Geometry: final body of the model. Coordinates: model frame, mm. A direction names the side the tool comes from. Give positions to 0.01 mm unless a question says otherwise; leave off trailing zeros. Write each loop counter-clockwise with the first axis right and the second up, starting at its lowest first coordinate (ties: lowest second). Pieces come first, ordered by that corner, then holes. Notation, with made-up numbers: (88, 0.5) - (119, 0.5) arc R21 ccw to (119, 25.5) - close; hole circle Ø8 at (36.5, -38.5). An arc over 180 degrees is marked (long way). Use CSV: the item, a comma, the result in double quotes. Start each with the question number.
(1) Section A-A on x = 6. Output: boundary loops of the cut face in (y, z), and give its area (3 significant figures).
(2) Reachability of faces 4 (the flat face through (10, 4, -10)), 5 (the flat face through (28.63, 3.45, -7.57)), 6 (the flat face through (28, 11, -10)) from +Z, -Z, +X, -X, +Y, -Y: full face, straight path, thin tool, end or side. Return the list, or none.
(3) Draft query along X for faces 1 (the flat face through (20, 0, -10)), 2 (the flat face through (20, 7, -10)), 3 (the flat face through (31.413, 3.451, -7.597)). Return one class per face: released by +X, released by -X, zero draft, split by the parting line, or undercut.
(4) Section B-B on y = 5.5. Output: boundary loops of the cut face in (x, z).
(5) Section C-C on z = -10. Output: boundary loops of the cut face in (x, y), and give its area (3 significant figures).
(6) Section D-D on y = 1.75. Output: boundary loops of the cut face in (x, z), and give its area (3 significant figures).
(7) Line query: probe 1 along X at (y, z) = (1.8, -10); probe 2 along X at (y, z) = (5, -10.5); probe 3 along Z at (x, y) = (6, 2.85). Output: solid intervals per line, ascending. Write a range as [from, to].
(8) First-contact query: pin 1 Ø1 at (y, z) = (6.5, -13) entering from -X; pin 2 Ø4.5 at (x, z) = (30, -10) entering from +Y; pin 3 Ø6 at (x, z) = (8.5, -11) entering from +Y; pin 4 Ø3 at (x, z) = (30.5, -11) entering from -Y. Flat tips, straight axial feed; report the tip coordinate or a pass-through.
from build123d import *

# Parameters (mm, degrees)
SKETCH1_W           = 40
SKETCH1_H           = 20
SKETCH1_R           = 2.75
BOSS_EXTRUDE1_DEPTH = 4
SKETCH2_W           = 20
SKETCH2_H           = 20
BOSS_EXTRUDE2_DEPTH = 7
SKETCH3_R           = 1.75
CUT_EXTRUDE1_DEPTH  = 12
CUT_EXTRUDE2_DEPTH  = 7


with BuildPart() as part:
    # Sketch1 → Boss-Extrude1 (new body)
    with BuildSketch(Plane(origin=(0, 0, 0), x_dir=(1, 0, 0), z_dir=(0, 1, 0))):
        with Locations((20, 10)):
            Rectangle(SKETCH1_W, SKETCH1_H)
        with Locations((6, 10)):
            Circle(SKETCH1_R, mode=Mode.SUBTRACT)
    extrude(amount=BOSS_EXTRUDE1_DEPTH)

    # Sketch2 → Boss-Extrude2 (add)
    with BuildSketch(Plane(origin=(0, 4, 0), x_dir=(1, 0, 0), z_dir=(0, 1, 0))):
        with Locations((30, 10)):
            Rectangle(SKETCH2_W, SKETCH2_H)
    extrude(amount=BOSS_EXTRUDE2_DEPTH)

    # Sketch3 → Cut-Extrude1 (cut, through all)
    with BuildSketch(Plane(origin=(0, 11, 0), x_dir=(1, 0, 0), z_dir=(0, 1, 0))):
        with Locations((30, 10)):
            Circle(SKETCH3_R)
    extrude(amount=-CUT_EXTRUDE1_DEPTH, mode=Mode.SUBTRACT)

    # Sketch4 → Cut-Extrude2 (cut)
    with BuildSketch(Plane(origin=(0, 0, 0), x_dir=(-1, 0, 0), z_dir=(0, -1, 0))):
        Polygon((-30, 13.218727751), (-32.7875, 11.609363875), (-32.7875, 8.390636125), (-30, 6.781272249), (-27.2125, 8.390636125), (-27.2125, 11.609363875), align=None)
    extrude(amount=-CUT_EXTRUDE2_DEPTH, mode=Mode.SUBTRACT)


solid = part.part
Check values:
1,outline,"(0, -20) - (4, -20) - (4, -12.75) - (0, -12.75) - close; (0, -7.25) - (4, -7.25) - (4, 0) - (0, 0) - close"
1,area,"58.0 mm²"
2,face 4,"+Z, -Z, -X, +Y"
2,face 5,"-Y"
2,face 6,"+Z, -Z, +X, -X, +Y"
3,face 1,"zero draft"
3,face 2,"released by -X"
3,face 3,"undercut"
4,outline,"(20, -20) - (40, -20) - (40, 0) - (20, 0) - close; hole (27.21, -11.61) - (30, -13.22) - (32.79, -11.61) - (32.79, -8.39) - (30, -6.78) - (27.21, -8.39) - close"
5,outline,"(0, 0) - (3.25, 0) - (3.25, 4) - (0, 4) - close; (8.75, 0) - (27.21, 0) - (27.21, 7) - (28.25, 7) - (28.25, 11) - (20, 11) - (20, 4) - (8.75, 4) - close; (31.75, 7) - (32.79, 7) - (32.79, 0) - (40, 0) - (40, 11) - (31.75, 11) - close"
5,area,"225 mm²"
6,outline,"(0, -20) - (40, -20) - (40, 0) - (0, 0) - close; hole circle Ø5.5 at (6, -10); hole (27.21, -11.61) - (30, -13.22) - (32.79, -11.61) - (32.79, -8.39) - (30, -6.78) - (27.21, -8.39) - close"
6,area,"749 mm²"
7,probe 1,"x = [0, 3.25], [8.75, 27.21], [32.79, 40]"
7,probe 2,"x = [20, 27.21], [32.79, 40]"
7,probe 3,"z = [-20, -12.75], [-7.25, 0]"
8,pin 1,"stops at x = 20"
8,pin 2,"stops at y = 11"
8,pin 3,"stops at y = 4"
8,pin 4,"stops at y = 7"
